from build123d import *

# Parameters (mm, degrees)
F0_W      = 50.8
F0_H      = 7.62
F1_DEPTH  = 7.62
F2_W      = 5.08
F2_H      = 7.62
F3_DEPTH  = 7.62
F4_R      = 2.54
F5_DEPTH  = 25.4
F6_W      = 22.86
F6_H      = 22.86
F6_W_2    = 7.62
F6_H_2    = 7.62
F7_DEPTH  = 50.8
F8_R      = 6.35
F8_R_2    = 3.81
F9_DEPTH  = 50.8
F10_W     = 50.8
F10_H     = 2.54
F11_DEPTH = 35.56
F12_W     = 2.54
F12_H     = 6.35
F12_W_2   = 15.24
F13_DEPTH = 6.35
F14_R     = 1.27
F15_DEPTH = 25.4
F16_W     = 2.54
F16_H     = 6.35
F16_W_2   = 15.24
F17_DEPTH = 6.35


with BuildPart() as f1:
    # F0 (on Right) → F1 (new body)
    with BuildSketch(Plane.YZ):
        with Locations((-27.0321643911, 33.6084578316)):
            Rectangle(F0_W, F0_H)
    extrude(amount=F1_DEPTH)

    # F2 (on face) → F3 (join)
    with BuildSketch(Plane.XZ.offset(52.4321643911)):
        with Locations((3.81, 33.6084578316)):
            Rectangle(F2_W, F2_H)
    extrude(amount=F3_DEPTH)

    # F4 (on face) → F5 (cut)
    with BuildSketch(Plane.YZ.offset(6.35)):
        with Locations((-56.2421643911, 33.6084578316)):
            Circle(F4_R)
        with BuildLine():
            ThreePointArc((-56.2421643911, 29.7984578316), (-59.9211503168, 33.6084578316), (-56.2421643911, 37.4184578316))
            Line((-56.2421643911, 37.4184578316), (-60.0521643911, 37.4184578316))
            Line((-60.0521643911, 37.4184578316), (-60.0521643911, 29.7984578316))
            Line((-60.0521643911, 29.7984578316), (-56.2421643911, 29.7984578316))
        make_face()
    extrude(amount=-F5_DEPTH, mode=Mode.SUBTRACT)

    # F6 (on face) → F7 (join)
    with BuildSketch(Plane(origin=(0, -1.6321643911, 0), x_dir=(-1, 0, 0), z_dir=(0, 1, 0))):
        with Locations((-3.81, 33.6136929691)):
            Rectangle(F6_W, F6_H)
        with Locations((-3.81, 33.6084578316)):
            Rectangle(F6_W_2, F6_H_2, mode=Mode.SUBTRACT)
        with Locations((-3.81, 33.6084578316)):
            Rectangle(F6_W_2, F6_H_2)
    extrude(amount=F7_DEPTH)

    # F8 (on face) → F9 (join)
    with BuildSketch(Plane(origin=(0, 49.1678356089, 0), x_dir=(-1, 0, 0), z_dir=(0, 1, 0))):
        with Locations((-3.81, 33.6136929691)):
            Circle(F8_R)
        with Locations((-3.81, 33.6136929691)):
            Circle(F8_R_2, mode=Mode.SUBTRACT)
    extrude(amount=F9_DEPTH)

    # F10 (on face) → F11 (join)
    with BuildSketch(Plane.YZ.offset(15.24)):
        with Locations((23.7678356089, 33.6136929691)):
            Rectangle(F10_W, F10_H)
    extrude(amount=-F11_DEPTH)

    # F12 (on face) → F13 (join)
    with BuildSketch(Plane(origin=(-7.62, 0, 0), x_dir=(0, -1, 0), z_dir=(-1, 0, 0))):
        with Locations((-35.1978356089, 38.0586929691)):
            Rectangle(F12_W, F12_H)
        with Locations((-23.7678356089, 38.0586929691)):
            Rectangle(F12_W_2, F12_H)
        with Locations((-12.3378356089, 38.0586929691)):
            Rectangle(F12_W, F12_H)
    extrude(amount=F13_DEPTH)

    # F14 (on face) → F15 (cut)
    with BuildSketch(Plane(origin=(0, 36.4678356089, 0), x_dir=(-1, 0, 0), z_dir=(0, 1, 0))):
        with Locations((10.795, 38.0586929691)):
            Circle(F14_R)
    extrude(amount=-F15_DEPTH, mode=Mode.SUBTRACT)

    # F16 (on face) → F17 (join)
    with BuildSketch(Plane(origin=(-7.62, 0, 0), x_dir=(0, -1, 0), z_dir=(-1, 0, 0))):
        with Locations((-35.1978356089, 29.1686929691)):
            Rectangle(F16_W, F16_H)
        with Locations((-23.7678356089, 29.1686929691)):
            Rectangle(F16_W_2, F16_H)
        with Locations((-12.3378356089, 29.1686929691)):
            Rectangle(F16_W, F16_H)
    extrude(amount=F17_DEPTH)


solid = f1.part
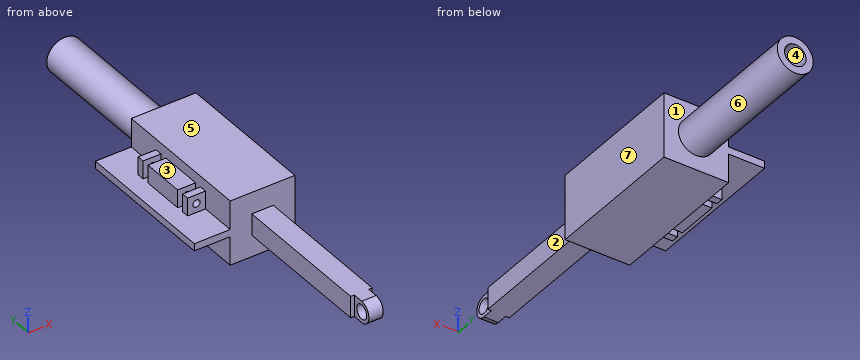
Here's how the part is built. I have some questions about the finished solid (model axes, mm). Face numbers are marked on the shaded views. A direction names the side the tool comes from. Round coordinates to 2 decimals unless told otherwise and drop trailing zeros. Loops run counter-clockwise (first coordinate to the right, second up) from the corner with the lowest first, then second, coordinate; pieces in that order, holes last. Notation, with made-up numbers: (52, -28.5) -> (97, -28.5) arc R32 cw to (97, -2.5) -> close; hole circle Ø2 at (86, 14.5). An arc over 180 degrees is marked (long way). Write each question's results on one line, items separated by ' | '.
(1) For the marked faces 1, 2 and 3, which set-ups out of +Z, -Z, +X, -X, +Y, -Y let a thin tool reach every point of the face, with its end or its side?
Worked answers:
face 1: +Y | face 2: +Z, -Z, +X, -Y | face 3: +Z, -X, +Y, -Y
(2) We'd pull the mould along X, two halves only. Please class the marked faces 4, 5, 6 and 7: released by +X, released by -X, zero draft, split by the parting line, or undercut.
Worked answers:
face 4: undercut | face 5: zero draft | face 6: split by the parting line | face 7: released by +X
(3) If we section it at C-C, the plane x = -4: List the corners of the cut face in (y, z) for me, then the cut area to 3 significant figures.
Worked answers:
outline: (-1.63, 22.18) -> (49.17, 22.18) -> (49.17, 45.04) -> (-1.63, 45.04) -> close | area: 1,160 mm2
(4) If I drill on L1, parallel to Y at x = -9.5, z = 35; L2, parallel to X at y = -46.5, z = 37; L3, parallel to X at y = 45, z = 30.5, over which ranges is the centre line in solid material (lowest first)?
Worked answers:
L1: 11.07 to 13.61, 16.15 to 31.39, 33.93 to 36.47 | L2: 0 to 7.62 | L3: -7.62 to 15.24
(5) If we section it at A-A, the plane x = 3.81: List the corners of the cut face in (y, z) for me.
Worked answers:
outline: (-56.24, 29.8) -> (-1.63, 29.8) -> (-1.63, 22.18) -> (49.17, 22.18) -> (49.17, 27.26) -> (99.97, 27.26) -> (99.97, 29.8) -> (49.17, 29.8) -> (49.17, 37.42) -> (99.97, 37.42) -> (99.97, 39.96) -> (49.17, 39.96) -> (49.17, 45.04) -> (-1.63, 45.04) -> (-1.63, 37.42) -> (-56.24, 37.42) arc R3.81 ccw to start; hole circle Ø5.08 at (-56.24, 33.61)
(6) If we section it at D-D, the plane y = 61.5: List the corners of the cut face in (x, z) for me.
Worked answers:
outline: circle Ø12.7 at (3.81, 33.61); hole circle Ø7.62 at (3.81, 33.61)
(7) For P1, Ø1.9, axis at x = -9.5, z = 28.5, coming from the -Y side; P2, Ø1.5, axis at x = -1.5, y = 62.5, coming from the +Z side; P3, Ø10, axis at x = 4, y = -35.5, coming from the -Z side, each with a flat end and sliding along its axis, tell me the tip position at first contact or that it passes through.
Worked answers:
P1: y = 11.07 | P2: z = 38.03 | P3: z = 29.8
(8) If we section it at B-B, the plane y = 1.5: List the corners of the cut face in (x, z) for me, then the cut area to 3 significant figures.
Worked answers:
outline: (-20.32, 32.34) -> (-7.62, 32.34) -> (-7.62, 22.18) -> (15.24, 22.18) -> (15.24, 45.04) -> (-7.62, 45.04) -> (-7.62, 34.88) -> (-20.32, 34.88) -> close | area: 555 mm2
